Check sheet for the modelled part. Datum: model origin and axes. Units: mm. A direction names the side the tool comes from. Round coordinates to 2 decimals unless told otherwise and drop trailing zeros. Write each loop counter-clockwise with the first axis right and the second up, starting at its lowest first coordinate (ties: lowest second). Pieces come first, ordered by that corner, then holes. Notation, with made-up numbers: M -21.75,14 L -11.75,14 A30 cw -11.75,38 Z; hole C 70,65 d4. An arc over 180 degrees is marked long. Put each result on its own line as item: value.
```python
from build123d import *

# Parameters (mm, degrees)
MODEL_R         = 1
MODEL_R_2       = 1.5
MODEL_R_3       = 1.2
MODEL_R_4       = 9.672061212
MODEL_W         = 5.108352415
MODEL_H         = 21
EXTRUDE_1_DEPTH = 1.6


with BuildPart() as part:
    # Model → 凸台-拉伸1 (new body)
    with BuildSketch(Plane.XY):
        with BuildLine():
            Line((164.249855651, 187.088781669), (146.787217515, 187.088781669))
            Line((146.787217515, 187.088781669), (129.32457938, 187.088781669))
            add(Edge.make_bspline(
                [(129.32457938, 187.088781669), (125.461044671, 187.088781669), (126.746381631, 178.375641151), (129.32457938, 175.498177543)],
                knots=[0, 0, 0, 0, 11.590604126, 11.590604126, 11.590604126, 11.590604126], degree=3))
            ThreePointArc((129.32457938, 175.498177543), (139.773420004, 147.014985412), (127.780187237, 119.146851779))
            ThreePointArc((127.780187237, 119.146851779), (118.967335725, 112.447515783), (108.683438965, 108.350087077))
            ThreePointArc((108.683438965, 108.350087077), (103.514701902, 100.139821501), (108.683438965, 91.929555925))
            ThreePointArc((108.683438965, 91.929555925), (118.967335725, 87.832127219), (127.780187237, 81.132791223))
            ThreePointArc((127.780187237, 81.132791223), (139.177354468, 59.195873616), (135.89135677, 34.694322764))
            add(Edge.make_bspline(
                [(135.89135677, 34.694322764), (132.800282497, 28.120921276), (160.774152533, 29.120921276), (157.683078261, 34.694322764)],
                knots=[0, 0, 0, 0, 21.791721492, 21.791721492, 21.791721492, 21.791721492], degree=3))
            ThreePointArc((157.683078261, 34.694322764), (154.397080563, 59.195873616), (165.794247794, 81.132791223))
            ThreePointArc((165.794247794, 81.132791223), (174.607099306, 87.832127219), (184.890996066, 91.929555925))
            ThreePointArc((184.890996066, 91.929555925), (190.059733129, 100.139821501), (184.890996066, 108.350087077))
            ThreePointArc((184.890996066, 108.350087077), (174.607099306, 112.447515783), (165.794247794, 119.146851779))
            ThreePointArc((165.794247794, 119.146851779), (153.801015027, 147.014985412), (164.249855651, 175.498177543))
            add(Edge.make_bspline(
                [(164.249855651, 187.088781669), (168.11339036, 187.088781669), (166.8280534, 178.375641151), (164.249855651, 175.498177543)],
                knots=[0, 0, 0, 0, 11.590604126, 11.590604126, 11.590604126, 11.590604126], degree=3))
        make_face()
        with Locations((156.787217515, 110.139821501)):
            Circle(MODEL_R, mode=Mode.SUBTRACT)
        with Locations((136.787217515, 110.139821501)):
            Circle(MODEL_R, mode=Mode.SUBTRACT)
        with Locations((136.787217515, 90.139821501)):
            Circle(MODEL_R, mode=Mode.SUBTRACT)
        with Locations((156.787217515, 90.139821501)):
            Circle(MODEL_R, mode=Mode.SUBTRACT)
        with Locations((168.353974342, 100.139821501)):
            Circle(MODEL_R_2, mode=Mode.SUBTRACT)
        with Locations((146.787217515, 121.706578327)):
            Circle(MODEL_R_2, mode=Mode.SUBTRACT)
        with Locations((125.220460689, 100.139821501)):
            Circle(MODEL_R_2, mode=Mode.SUBTRACT)
        with Locations((146.787217515, 78.573064675)):
            Circle(MODEL_R_2, mode=Mode.SUBTRACT)
        with Locations((146.787217515, 126.706578327)):
            Circle(MODEL_R_2, mode=Mode.SUBTRACT)
        with Locations((120.220460689, 100.139821501)):
            Circle(MODEL_R_2, mode=Mode.SUBTRACT)
        with Locations((146.787217515, 73.573064675)):
            Circle(MODEL_R_2, mode=Mode.SUBTRACT)
        with Locations((173.353974342, 100.139821501)):
            Circle(MODEL_R_2, mode=Mode.SUBTRACT)
        with Locations((146.787217515, 118.171044401)):
            Circle(MODEL_R, mode=Mode.SUBTRACT)
        with Locations((128.755994615, 100.139821501)):
            Circle(MODEL_R, mode=Mode.SUBTRACT)
        with Locations((146.787217515, 82.108598601)):
            Circle(MODEL_R, mode=Mode.SUBTRACT)
        with Locations((164.818440415, 100.139821501)):
            Circle(MODEL_R, mode=Mode.SUBTRACT)
        with Locations((162.037217515, 115.389821501)):
            Circle(MODEL_R_2, mode=Mode.SUBTRACT)
        with Locations((131.537217515, 115.389821501)):
            Circle(MODEL_R_2, mode=Mode.SUBTRACT)
        with Locations((131.537217515, 84.889821501)):
            Circle(MODEL_R_2, mode=Mode.SUBTRACT)
        with Locations((162.037217515, 84.889821501)):
            Circle(MODEL_R_2, mode=Mode.SUBTRACT)
        with Locations((182.657217515, 100.139821501)):
            Circle(MODEL_R, mode=Mode.SUBTRACT)
        with Locations((146.787217515, 136.036864466)):
            Circle(MODEL_R, mode=Mode.SUBTRACT)
        with Locations((110.917217515, 100.139821501)):
            Circle(MODEL_R, mode=Mode.SUBTRACT)
        with Locations((146.787217515, 64.242778536)):
            Circle(MODEL_R, mode=Mode.SUBTRACT)
        with Locations((146.787217515, 36.419821501)):
            Circle(MODEL_R, mode=Mode.SUBTRACT)
        with Locations((158.787217515, 182.099821501)):
            Circle(MODEL_R, mode=Mode.SUBTRACT)
        with Locations((134.787217515, 182.099821501)):
            Circle(MODEL_R, mode=Mode.SUBTRACT)
        with Locations((128.00168361, 111.854287595)):
            Circle(MODEL_R_3, mode=Mode.SUBTRACT)
        with Locations((165.572751421, 111.854287595)):
            Circle(MODEL_R_3, mode=Mode.SUBTRACT)
        with Locations((128.00168361, 88.425355407)):
            Circle(MODEL_R_3, mode=Mode.SUBTRACT)
        with Locations((165.572751421, 88.425355407)):
            Circle(MODEL_R_3, mode=Mode.SUBTRACT)
        with Locations((146.787217515, 100.139821501)):
            Circle(MODEL_R_4, mode=Mode.SUBTRACT)
        with BuildLine():
            Line((159.067032454, 178.883153661), (146.787217515, 178.883153661))
            Line((146.787217515, 178.883153661), (134.507402577, 178.883153661))
            add(Edge.make_bspline(
                [(134.507402577, 178.883153661), (133.227688428, 178.883153661), (133.453062144, 176.072728685), (134.227836458, 175.05420374)],
                knots=[0, 0, 0, 0, 3.839142445, 3.839142445, 3.839142445, 3.839142445], degree=3))
            ThreePointArc((134.227836458, 175.05420374), (142.088179874, 158.46992126), (142.587324671, 140.123960438))
            add(Edge.make_bspline(
                [(142.587324671, 140.123960438), (142.493407811, 139.609308925), (142.9625841, 138.837088874), (143.485734707, 138.837088874)],
                knots=[0, 0, 0, 0, 1.56945182, 1.56945182, 1.56945182, 1.56945182], degree=3))
            Line((143.485734707, 138.837088874), (146.787217515, 138.837088874))
            Line((146.787217515, 138.837088874), (150.088700324, 138.837088874))
            add(Edge.make_bspline(
                [(150.98711036, 140.123960438), (151.08102722, 139.609308925), (150.611850931, 138.837088874), (150.088700324, 138.837088874)],
                knots=[0, 0, 0, 0, 1.56945182, 1.56945182, 1.56945182, 1.56945182], degree=3))
            ThreePointArc((150.98711036, 140.123960438), (151.486255157, 158.46992126), (159.346598573, 175.05420374))
            add(Edge.make_bspline(
                [(159.067032454, 178.883153661), (160.346746603, 178.883153661), (160.121372887, 176.072728685), (159.346598573, 175.05420374)],
                knots=[0, 0, 0, 0, 3.839142445, 3.839142445, 3.839142445, 3.839142445], degree=3))
        make_face(mode=Mode.SUBTRACT)
        with BuildLine():
            Line((151.053210178, 121.070269245), (157.209188782, 121.070269245))
            add(Edge.make_bspline(
                [(157.209188782, 121.070269245), (158.876955289, 121.070269245), (158.876955289, 116.066969722), (157.209188782, 116.066969722)],
                knots=[0, 0, 0, 0, 5.003299523, 5.003299523, 5.003299523, 5.003299523], degree=3))
            Line((157.209188782, 116.066969722), (151.053210178, 116.066969722))
            add(Edge.make_bspline(
                [(151.053210178, 121.070269245), (149.38544367, 121.070269245), (149.38544367, 116.066969722), (151.053210178, 116.066969722)],
                knots=[0, 0, 0, 0, 5.003299523, 5.003299523, 5.003299523, 5.003299523], degree=3))
        make_face(mode=Mode.SUBTRACT)
        with BuildLine():
            Line((136.47001729, 84.090392193), (142.625995894, 84.090392193))
            add(Edge.make_bspline(
                [(142.625995894, 84.090392193), (144.706817358, 84.090392193), (144.706817358, 77.847927799), (142.625995894, 77.847927799)],
                knots=[0, 0, 0, 0, 6.242464394, 6.242464394, 6.242464394, 6.242464394], degree=3))
            Line((142.625995894, 77.847927799), (136.47001729, 77.847927799))
            add(Edge.make_bspline(
                [(136.47001729, 84.090392193), (134.389195825, 84.090392193), (134.389195825, 77.847927799), (136.47001729, 77.847927799)],
                knots=[0, 0, 0, 0, 6.242464394, 6.242464394, 6.242464394, 6.242464394], degree=3))
        make_face(mode=Mode.SUBTRACT)
        with BuildLine():
            Line((139.974283877, 181.317718414), (153.600151154, 181.317718414))
            add(Edge.make_bspline(
                [(153.600151154, 184.631261375), (154.704665474, 184.631261375), (154.704665474, 181.317718414), (153.600151154, 181.317718414)],
                knots=[0, 0, 0, 0, 3.313542961, 3.313542961, 3.313542961, 3.313542961], degree=3))
            Line((153.600151154, 184.631261375), (139.974283877, 184.631261375))
            add(Edge.make_bspline(
                [(139.974283877, 184.631261375), (138.869769557, 184.631261375), (138.869769557, 181.317718414), (139.974283877, 181.317718414)],
                knots=[0, 0, 0, 0, 3.313542961, 3.313542961, 3.313542961, 3.313542961], degree=3))
        make_face(mode=Mode.SUBTRACT)
        with Locations((146.787217516, 50.217854956)):
            Rectangle(MODEL_W, MODEL_H, mode=Mode.SUBTRACT)
    extrude(amount=EXTRUDE_1_DEPTH)


solid = part.part
```
1. Cross-section at A-A (y = 162.5). Enter the section's corners in (x, z).
Computed values:
outline: M 137.19,0 L 140.92,0 L 140.92,1.6 L 137.19,1.6 Z; M 152.65,0 L 156.38,0 L 156.38,1.6 L 152.65,1.6 Z
2. Scan lines: probe 1 along Y at (x, z) = (161.5, 0.1); probe 2 along Y at (x, z) = (143.5, 0.6); probe 3 along X at (y, z) = (89.5, 0.2). Record each from-to range of solid material in increasing order.
Computed values:
probe 1: y = 76.08 to 83.49, 86.29 to 113.99, 116.79 to 124.2, 172.08 to 187.09
probe 2: y = 30.22 to 78.32, 83.62 to 91.04, 109.24 to 138.84, 178.88 to 181.32, 184.63 to 187.09
probe 3: x = 115.68 to 127.47, 128.54 to 136.02, 137.56 to 156.02, 157.56 to 165.04, 166.11 to 177.89
3. Access from +Z, -Z, +X, -X, +Y, -Y to the whole of each face (thin tool, end or side, straight path). Record for faces 1 (the cylindrical face through (151.427, 158.218, 0.789)), 2 (the cylindrical face through (190.06, 100, 0.79)).
Computed values:
face 1: +Z, -Z
face 2: +Z, -Z, +X
4. Cross-section at D-D (y = 131.5). Enter the section's corners in (x, z), then the cut area to 3 significant figures.
Computed values:
outline: M 136.26,0 L 157.31,0 L 157.31,1.6 L 136.26,1.6 Z
area: 33.7 mm2
5. Cross-section at C-C (y = 70). Enter the section's corners in (x, z).
Computed values:
outline: M 135.7,0 L 157.88,0 L 157.88,1.6 L 135.7,1.6 Z
6. Cross-section at B-B (z = 0.4). Count the separate pieces of the cut face and the enclosed holes in it, then the cut area to 3 significant figures.
Computed values:
separate pieces: 1
enclosed holes: 37
area: 3,940 mm2
7. Release check for a two-part mould opening along X. For faces 3 (the flat face through (140, 108, 0)), 4 (the cylindrical face through (103.516, 100.283, 0.789)), 5 (the cylindrical face through (148.173, 77.999, 0.789)) record: +X half, -X half, draft (parallel to the pull), parting line (faces both ways), or undercut.
Computed values:
face 3: draft
face 4: -X half
face 5: undercut
